Autodesk Inventor part; units mm, degrees
ref_plane "YZ Plane" through (0, 0, 0) normal (1, 0, 0) x (0, 1, 0)
ref_plane "XZ Plane" through (0, 0, 0) normal (0, 1, 0) x (-1, 0, 0)
ref_plane "XY Plane" through (0, 0, 0) normal (0, 0, 1) x (1, 0, 0)
sketch "Esquisse1" plane through (0, 0, 0) normal (0, 0, 1) x (1, 0, 0)
  line L0 (4.94, 2.8521) -> (4.94, -2.8521)
  line L1 (4.94, -2.8521) -> (0, -5.7042)
  line L2 (0, -5.7042) -> (-4.94, -2.8521)
  line L3 (-4.94, -2.8521) -> (-4.94, 2.8521)
  line L4 (-4.94, 2.8521) -> (0, 5.7042)
  line L5 (0, 5.7042) -> (4.94, 2.8521)
  point P0 (0, 0)
  point P1 (0, 0)
  dimension "d0" = 9.88
extrude "Extrusion1" add sketch "Esquisse1" along normal mid plane 1.96
sketch "Esquisse2" plane through (0, 0, 0.98) normal (0, 0, 1) x (1, 0, 0)
  point P0 (0, 0)
  point P1 (0, 0)
hole "Perçage1" at (0, 0, 0.98) direction (0, 0, -1) diameter 7.459 depth 18.8 tip angle 118
sketch "Esquisse3" plane through (0, 0, 0) normal (0, 1, 0) x (-1, 0, 0)
  line L0 (-4.94, 0.98) -> (0, 0.98) construction
  line L1 (-4.94, -0.98) -> (-4.94, 0.98) construction
  line L2 (-3.94, 1.93) -> (-5.94, -0.07)
  line L3 (-5.94, -0.07) -> (-5.94, 1.93)
  line L4 (-5.94, 1.93) -> (-3.94, 1.93)
  line L5 (0, -1.432) -> (0, 1.732)
  point P0 (0, 0)
  point P1 (-4.89, 0.98)
  point P2 (-4.94, 0.93)
  point P3 (-4.94, 1.93)
  dimension "d12" = 0.05
  dimension "d13" = 0.05
  dimension "d14" = 2
revolve "Révolution1" cut sketch "Esquisse3" angle 360 about axis through (0, 0, -10) along (0, 0, 1)
mirror "Symétrie1" about plane through (0, 0, 0) normal (0, 0, 1) of "Révolution1"
properties part number "Ecrou plug alimentation" material "----------"
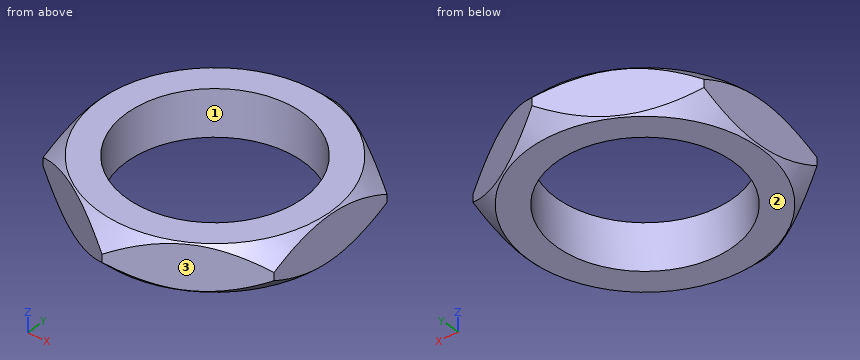
Check sheet for the modelled part. Datum: model origin and axes. Units: mm. Face numbers are marked on the shaded views. Round coordinates to 2 decimals unless told otherwise and drop trailing zeros. Loops run counter-clockwise (first coordinate to the right, second up) from the corner with the lowest first, then second, coordinate; pieces in that order, holes last.
1. Sectioned sample at C-C on z = 0.35. Record the boundary of the cut face in (x, y), and give its area (3 significant figures).
2. Sectioned sample at B-B on z = -0.6. Record the boundary of the cut face in (x, y), and give its area (3 significant figures).
3. Gauge pin test, flat ends, axial feed: pin 1 Ø1.5 at (x, y) = (1, -3.5) entering from -Z; pin 2 Ø4.5 at (x, y) = (0, 0) entering from -Z. Record the tip position at first contact, or that the pin passes through.
4. Scan lines: probe 1 along X at (y, z) = (0, 0); probe 2 along X at (y, z) = (3, 0.65); probe 3 along Y at (x, z) = (-4.25, -0.75). Record each from-to range of solid material in increasing order.
5. Sectioned sample at A-A on y = 0. Record the boundary of the cut face in (x, z).
6. Mould release check, pull along X, two halves, no side actions. Record for the marked faces 1, 2 and 3: released by +X, released by -X, zero draft, split by the parting line, or undercut.
Recorded:
1. outline: (-4.94, -2.46) arc R5.52 ccw to (-4.6, -3.05) - (-0.34, -5.51) arc R5.52 ccw to (0.34, -5.51) - (4.6, -3.05) arc R5.52 ccw to (4.94, -2.46) - (4.94, 2.46) arc R5.52 ccw to (4.6, 3.05) - (0.34, 5.51) arc R5.52 ccw to (-0.34, 5.51) - (-4.6, 3.05) arc R5.52 ccw to (-4.94, 2.46) - close; hole circle Ø7.46 at (0, 0)
1. area: 40.5 mm2
2. outline: (-4.94, -1.84) arc R5.27 ccw to (-4.06, -3.36) - (-0.88, -5.2) arc R5.27 ccw to (0.88, -5.2) - (4.06, -3.36) arc R5.27 ccw to (4.94, -1.84) - (4.94, 1.84) arc R5.27 ccw to (4.06, 3.36) - (0.88, 5.2) arc R5.27 ccw to (-0.88, 5.2) - (-4.06, 3.36) arc R5.27 ccw to (-4.94, 1.84) - close; hole circle Ø7.46 at (0, 0)
2. area: 38.7 mm2
3. pin 1: stops at z = -0.98
3. pin 2: passes through
4. probe 1: x = -4.94 to -3.73, 3.73 to 4.94
4. probe 2: x = -4.27 to -2.22, 2.22 to 4.27
4. probe 3: y = -2.86 to 2.86
5. outline: (-4.94, -0.93) - (-4.89, -0.98) - (-3.73, -0.98) - (-3.73, 0.98) - (-4.89, 0.98) - (-4.94, 0.93) - close; (3.73, -0.98) - (4.89, -0.98) - (4.94, -0.93) - (4.94, 0.93) - (4.89, 0.98) - (3.73, 0.98) - close
6. face 1: undercut
6. face 2: zero draft
6. face 3: released by +X
